```python
from build123d import *

# Parameters (mm, degrees)
SKETCH_1_W           = 24
SKETCH_1_H           = 36
EXTRUDE_1_DEPTH      = 19
CUT_EXTRUDE_2_DEPTH  = 3.5
SKETCH_4_W           = 5.4
SKETCH_4_H           = 7
CUT_EXTRUDE_3_DEPTH  = 36.510561809
CUT_EXTRUDE_4_DEPTH  = 3.5
SKETCH_6_R           = 4.15
CUT_EXTRUDE_5_DEPTH  = 44.726422218
FILLET_2_R           = 3
SKETCH_10_W          = 10
SKETCH_10_H          = 36
CUT_EXTRUDE_9_DEPTH  = 36.510561809
SKETCH_11_W          = 28
SKETCH_11_H          = 16.5
EXTRUDE_3_DEPTH      = 24
SKETCH_12_W          = 10.25
SKETCH_12_H          = 12
EXTRUDE_4_DEPTH      = 7
FILLET_3_R           = 3.5
SKETCH_13_W          = 10.25
SKETCH_13_H          = 1.5
EXTRUDE_5_DEPTH      = 7
FILLET_4_R           = 3.5
SKETCH_14_R          = 5.6
CUT_EXTRUDE_10_DEPTH = 7
FILLET_6_R           = 3
EXTRUDE_START        = -18
SKETCH_16_R          = 4.15
EXTRUDE_6_DEPTH      = 18
SKETCH_18_R          = 7.65
SKETCH_18_W          = 28
SKETCH_18_H          = 9
SKETCH_18_H_2        = 17.5
CUT_EXTRUDE_11_DEPTH = 47.122120558
FILLET_7_R           = 8
SKETCH_19_R          = 1.5
CUT_EXTRUDE_12_DEPTH = 26
SKETCH_20_R          = 1.5
CUT_EXTRUDE_13_DEPTH = 20
SKETCH_21_R          = 2.5
CUT_EXTRUDE_14_DEPTH = 1


with BuildPart() as part:
    # 草图1 → 凸台-拉伸1 (new, symmetric)
    with BuildSketch(Plane.XY):
        Rectangle(SKETCH_1_W, SKETCH_1_H)
    extrude(amount=EXTRUDE_1_DEPTH, both=True)

    # 草图3 → 切除-拉伸2 (cut, symmetric)
    with BuildSketch(Plane(origin=(0, 3.5, 0), x_dir=(1, 0, 0), z_dir=(0, 1, 0))):
        with BuildLine():
            Line((-5.75, -7.5), (-12, -7.5))
            Line((-12, -7.5), (-12, 19))
            Line((-12, 19), (1.75, 19))
            Line((1.75, 19), (1.75, 0))
            ThreePointArc((1.75, 0), (-0.446699141, -5.303300859), (-5.75, -7.5))
        make_face()
    extrude(amount=CUT_EXTRUDE_2_DEPTH, both=True, mode=Mode.SUBTRACT)

    # 草图4 → 切除-拉伸3 (cut, through all)
    with BuildSketch(Plane.ZY.offset(12)):
        with Locations((4.8, -3.5)):
            Rectangle(SKETCH_4_W, SKETCH_4_H)
    extrude(amount=-CUT_EXTRUDE_3_DEPTH, mode=Mode.SUBTRACT)

    # 草图5 → 切除-拉伸4 (cut, symmetric)
    with BuildSketch(Plane(origin=(0, -3.5, 0), x_dir=(1, 0, 0), z_dir=(0, 1, 0))):
        with BuildLine():
            Line((5.75, 4), (12, 4))
            Line((12, 4), (12, 19))
            Line((12, 19), (-1.75, 19))
            Line((-1.75, 19), (-1.75, 11.5))
            ThreePointArc((-1.75, 11.5), (0.446699141, 6.196699141), (5.75, 4))
        make_face()
    extrude(amount=CUT_EXTRUDE_4_DEPTH, both=True, mode=Mode.SUBTRACT)

    # 草图6 → 切除-拉伸5 (cut, through all)
    with BuildSketch(Plane(origin=(0, 0, -19), x_dir=(-1, 0, 0), z_dir=(0, 0, -1))):
        with Locations((0, 12)):
            Circle(SKETCH_6_R)
        with Locations(Location((0, -12, 0), (0, 0, 180))):
            Circle(SKETCH_6_R)
    extrude(amount=-CUT_EXTRUDE_5_DEPTH, mode=Mode.SUBTRACT)

    # 圆角2
    fillet_2_edges = [part.edges().sort_by_distance(p)[0] for p in [
        (6.725, 0, 2.1),
        (0, -7, 2.1),
    ]]
    fillet(fillet_2_edges, radius=FILLET_2_R)

    # 草图10 → 切除-拉伸9 (cut, through all)
    with BuildSketch(Plane(origin=(12, 0, 0), x_dir=(0, 0, -1), z_dir=(1, 0, 0))):
        with Locations((-14, 0)):
            Rectangle(SKETCH_10_W, SKETCH_10_H)
    extrude(amount=-CUT_EXTRUDE_9_DEPTH, mode=Mode.SUBTRACT)

    # 草图11 → 凸台-拉伸3 (add)
    with BuildSketch(Plane.ZY.offset(12)):
        with Locations((-5, -26.25)):
            Rectangle(SKETCH_11_W, SKETCH_11_H)
    extrude_3 = extrude(amount=-EXTRUDE_3_DEPTH)

    # 镜向2: 凸台-拉伸3 across plane
    add(extrude_3.mirror(Plane.ZX))

    # 草图12 → 凸台-拉伸4 (add)
    with BuildSketch(Plane(origin=(0, 0, 0), x_dir=(1, 0, 0), z_dir=(0, 1, 0))):
        with Locations((-6.875, 13)):
            Rectangle(SKETCH_12_W, SKETCH_12_H)
    extrude(amount=EXTRUDE_4_DEPTH)

    # 圆角3
    fillet_3_edges = [part.edges().sort_by_distance(p)[0] for p in [
        (-6.875, 0, -7),
        (-6.875, 7, -7),
    ]]
    fillet(fillet_3_edges, radius=FILLET_3_R - 0.0001)  # a hair under: the kernel refuses the full size

    # 草图13 → 凸台-拉伸5 (add)
    with BuildSketch(Plane.XZ):
        with Locations((6.875, -18.25)):
            Rectangle(SKETCH_13_W, SKETCH_13_H)
    extrude(amount=EXTRUDE_5_DEPTH)

    # 圆角4
    fillet_4_edges = [part.edges().sort_by_distance(p)[0] for p in [
        (6.875, 0, -17.5),
        (6.875, -7, -17.5),
    ]]
    fillet(fillet_4_edges, radius=FILLET_4_R - 0.0001)  # a hair under: the kernel refuses the full size

    # 草图14 → 切除-拉伸10 (cut)
    with BuildSketch(Plane.XZ):
        with Locations((5.75, -11.5)):
            Circle(SKETCH_14_R)
    extrude(amount=CUT_EXTRUDE_10_DEPTH, mode=Mode.SUBTRACT)

    # 圆角6
    fillet_6_edges = [part.edges().sort_by_distance(p)[0] for p in [
        (-5.275, 0, 2.1),
    ]]
    fillet(fillet_6_edges, radius=FILLET_6_R)

    # 草图16 → 凸台-拉伸6 (add)
    with BuildSketch(Plane.XY.offset(9).offset(EXTRUDE_START)):
        with Locations((0, -12)):
            Circle(SKETCH_16_R)
        with Locations(Location((0, 12, 0), (0, 0, 180))):
            Circle(SKETCH_16_R)
    extrude(amount=EXTRUDE_6_DEPTH)

    # 草图18 → 切除-拉伸11 (cut, through all)
    with BuildSketch(Plane.ZY.offset(12)):
        with Locations(Location((0, -15.5, 0), (0, 0, 270))):
            Circle(SKETCH_18_R)
        with Locations((-5, -30)):
            Rectangle(SKETCH_18_W, SKETCH_18_H)
        with Locations((-5, 25.75)):
            Rectangle(SKETCH_18_W, SKETCH_18_H_2)
    extrude(amount=-CUT_EXTRUDE_11_DEPTH, mode=Mode.SUBTRACT)

    # 圆角7
    fillet_7_edges = [part.edges().sort_by_distance(p)[0] for p in [
        (12, 17, -5),
        (-12, 17, -5),
    ]]
    fillet(fillet_7_edges, radius=FILLET_7_R)

    # 草图19 → 切除-拉伸12 (cut)
    with BuildSketch(Plane(origin=(0, 17, 0), x_dir=(1, 0, 0), z_dir=(0, 1, 0))):
        with Locations(Location((5.75, 11.5, 0), (0, 0, 180))):
            Circle(SKETCH_19_R)
    extrude(amount=-CUT_EXTRUDE_12_DEPTH, mode=Mode.SUBTRACT)

    # 草图20 → 切除-拉伸13 (cut)
    with BuildSketch(Plane(origin=(0, 17, 0), x_dir=(1, 0, 0), z_dir=(0, 1, 0))):
        with Locations(Location((-5.75, 0, 0), (0, 0, 180))):
            Circle(SKETCH_20_R)
    extrude(amount=-CUT_EXTRUDE_13_DEPTH, mode=Mode.SUBTRACT)

    # 草图21 → 切除-拉伸14 (cut)
    with BuildSketch(Plane(origin=(0, 17, 0), x_dir=(1, 0, 0), z_dir=(0, 1, 0))):
        with Locations((5.75, 11.5)):
            Circle(SKETCH_21_R)
        with Locations((-5.75, 0)):
            Circle(SKETCH_21_R)
    extrude(amount=-CUT_EXTRUDE_14_DEPTH, mode=Mode.SUBTRACT)


solid = part.part
```
Model file for the job. Use its own axes, mm. A direction names the side the tool comes from. Give positions to 0.01 mm unless a question says otherwise; leave off trailing zeros. Loops run counter-clockwise (first coordinate to the right, second up) from the corner with the lowest first, then second, coordinate; pieces in that order, holes last. Notation, with made-up numbers: (-20, 0.25) -> (-1, 0.25) arc R24 cw to (-1, 19.25) -> close; hole circle Ø7 at (78.5, 46.25). An arc over 180 degrees is marked (long way). Use CSV: the item, a comma, the result in double quotes. Start each with the question number.
1) Wall check: line 1 (Z direction, x = -5.75, y = 14); line 2 (Z direction, x = -9.25, y = -5.5); line 3 (Y direction, x = -8, z = -0.25). Give the ranges that are in metal, low to high.
2) Slice it at B-B on z = 6.25. Give the cut face in (x, y).
3) Mould opens along X. For faces 6 (the cylindrical face through (5.366, -0.716, -17.087)), 7 (the cylindrical face through (-9.719, 14.594, -4.804)), 8 (the cylindrical face through (5.96, -0.9, 2.96)) say: released by +X, released by -X, zero draft, split by the parting line, or undercut.
4) Tool access for faces 1 (the cylindrical face through (0.17, -6.1, 2.96)), 2 (the flat face through (0, 12, -9)), 3 (the flat face through (0, -4, 9)), 4 (the flat face through (9, -3, -4)), 5 (the flat face through (-4, 16, 0)): list every direction of +Z, -Z, +X, -X, +Y, -Y with a clear straight run to the whole face (end or side of a thin tool).
5) Slice it at A-A on z = -11. Give the number of separate pieces and of enclosed holes in the cut face, plus the area to 3 significant figures.
6) Slice it at D-D on z = -16. Give the cut face in (x, y).
7) Slice it at C-C on y = 12. Give the cut face in (x, z), plus the area to 3 significant figures.
8) Flat gauge pin, fed straight in: pin 1 Ø1.9 at (x, z) = (-5, 7) entering from +Y. Where does the tip first touch, or does it go through?
Computed values:
1,line 1,"z = -19 to -1.5, 1.5 to 9"
1,line 2,"z = -19 to 2.5, 7.5 to 9"
1,line 3,"y = -25.5 to -23.15, -7.85 to -0.07, 7 to 15.93"
2,outline,"(-12, -25.5) -> (12, -25.5) -> (12, -19.91) -> (-12, -19.91) -> close; (-12, -11.09) -> (12, -11.09) -> (12, -7) -> (-12, -7) -> close; (-12, 7) -> (-1.6, 7) -> (-1.6, 0) -> (12, 0) -> (12, 9) arc R8 ccw to (4, 17) -> (-4, 17) arc R8 ccw to (-12, 9) -> close"
3,face 6,"undercut"
3,face 7,"released by -X"
3,face 8,"zero draft"
4,face 1,"+X, -X"
4,face 2,"-Z"
4,face 3,"+Z, +X, -X, +Y, -Y"
4,face 4,"+X"
4,face 5,"+Y"
5,separate pieces,"2"
5,enclosed holes,"2"
5,area,"709 mm^2"
6,outline,"(-12, -25.5) -> (12, -25.5) -> (12, -6.37) -> (9.08, -6.37) -> (9.08, -7) -> (2.42, -7) -> (2.42, -6.37) -> (1.75, -6.37) -> (1.75, -7) -> (-1.75, -7) -> (-1.75, 7) -> (1.75, 7) -> (1.75, -0.63) -> (2.42, -0.63) -> (2.42, 0) -> (9.08, 0) -> (9.08, -0.63) -> (12, -0.63) -> (12, 9) arc R8 ccw to (4, 17) -> (-4, 17) arc R8 ccw to (-12, 9) -> close; hole circle Ø8.3 at (0, -12); hole circle Ø8.3 at (0, 12)"
7,outline,"(-11.42, -19) -> (-4.15, -19) -> (-4.15, -9) -> (4.15, -9) -> (4.15, -19) -> (11.42, -19) -> (11.42, 9) -> (-11.42, 9) -> close; hole circle Ø3 at (-5.75, 0); hole circle Ø3 at (5.75, -11.5)"
7,area,"542 mm^2"
8,pin 1,"stops at y = 17"
